The figure shows three views and two pictorial views of one solid part (mm, origin at its lowest corner). Answer the questions. A direction names the side the tool comes from. Coordinates: 2 decimals unless noted, no trailing zeros. Write each loop counter-clockwise with the first axis right and the second up, starting at its lowest first coordinate (ties: lowest second). Pieces come first, ordered by that corner, then holes. Notation, with made-up numbers: M 75.25,-17.75 L 96.25,-17.75 A25 cw 96.25,1.25 Z; hole C -4,-28.5 d7. An arc over 180 degrees is marked long. Write item = value, one per line.
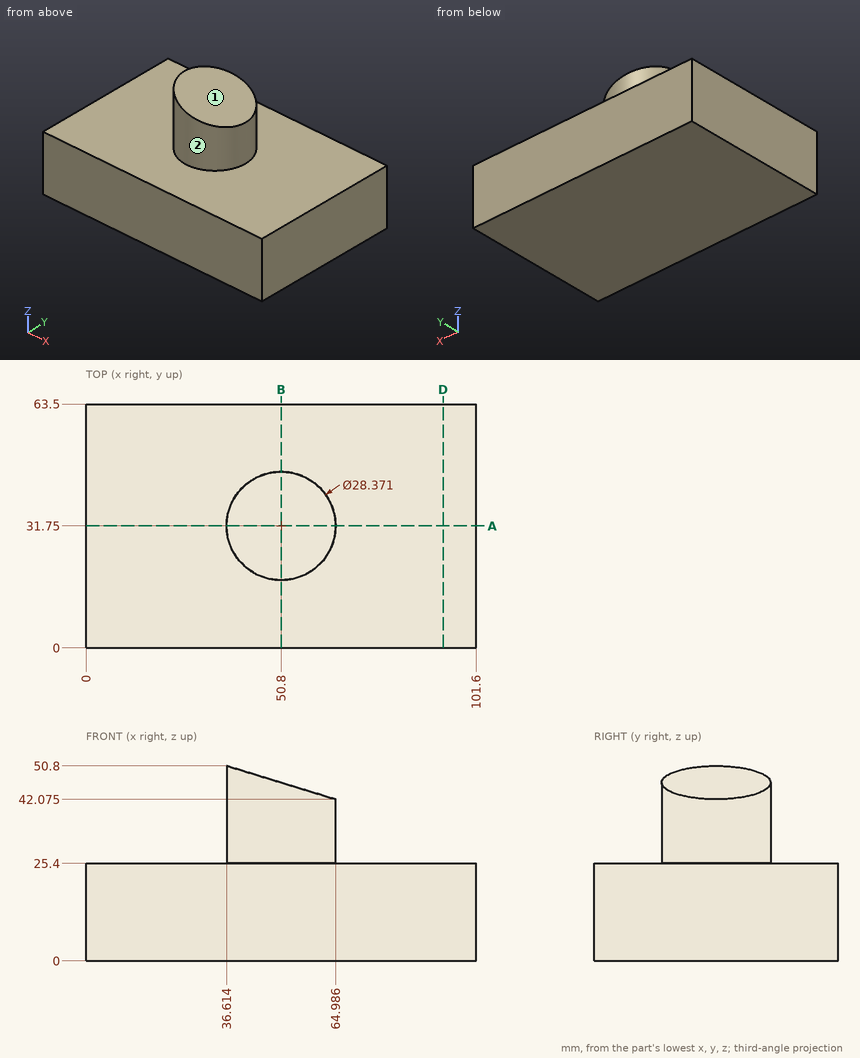
Item 1: Find section D-D (x = 93). Determine the outline of the cut face in (y, z), and give its area (3 significant figures).
Worked answers:
outline = M 0,0 L 63.5,0 L 63.5,25.4 L 0,25.4 Z
area = 1,610 mm²
Item 2: Flat-ended cylindrical pins translate along their axes: pin 1 (5 mm diameter, centred on y = 29.5, z = 41, fed in from -X); pin 2 (1.5 mm diameter, centred on y = 37.5, z = 35, fed in from -X) (1 decimal); pin 3 (19 mm diameter, centred on x = 59.5, y = 32, fed in from +Z). Find the tip coordinate at first contact, or state that the pin passes through.
Worked answers:
pin_1 = 36.61
pin_2 = 37.5
pin_3 = 46.68
Item 3: Find section A-A (y = 31.75). Determine the outline of the cut face in (x, z) (1 decimal), and give its area (3 significant figures).
Worked answers:
outline = M 0,0 L 101.6,0 L 101.6,25.4 L 65,25.4 L 65,42.1 L 36.6,50.8 L 36.6,25.4 L 0,25.4 Z
area = 3,180 mm²
Item 4: Consider line 1 along Z through (x, y) = (39.5, 56); line 2 along Y through (x, z) = (51, 43.5); line 3 along Z through (x, y) = (55.5, 21.5). Determine where each line is inside the solid, lowest interval first. Write a range as from..to.
Worked answers:
line_1 = 0..25.4
line_2 = 17.57..45.93
line_3 = 0..44.99
Item 5: Which of the six approach directions +Z, -Z, +X, -X, +Y, -Y give full straight-line access (tool end or side, diameter ignored) to the marked faces 1 and 2?
Worked answers:
face_1 = +Z, +X, +Y, -Y
face_2 = +Z
Item 6: Find section B-B (x = 50.8). Determine the outline of the cut face in (y, z) (1 decimal).
Worked answers:
outline = M 0,0 L 63.5,0 L 63.5,25.4 L 45.9,25.4 L 45.9,46.4 L 17.6,46.4 L 17.6,25.4 L 0,25.4 Z
